Design review of the part built by this model. Coordinates are the model's own, in mm. A direction names the side the tool comes from. Round coordinates to 2 decimals unless told otherwise and drop trailing zeros. Loops run counter-clockwise (first coordinate to the right, second up) from the corner with the lowest first, then second, coordinate; pieces in that order, holes last. Notation, with made-up numbers: M -36.75,81.5 L -3.75,81.5 A31 cw -3.75,107.5 Z; hole C 86,42 d10. An arc over 180 degrees is marked long. One line per item, written item: value. Start each with the question number.
Item 1: For line 1 along X through (y, z) = (1.4, 9); line 2 along Z through (x, y) = (12, 1.55); line 3 along Y through (x, z) = (0, 0.5), list the stretches that pass through material, from the lowest coordinate up.
Item 2: Mouldability with a two-part tool opening along Z and no side actions: class faces 6 (the flat face through (2, 24, -7.75)), 7 (the cylindrical face through (0.35, 8.94, -2.7)), 8 (the cylindrical face through (-13.08, 0.99, -10.18)), 9 (the flat face through (0, 1, 15)) as released by +Z, released by -Z, zero draft, split by the parting line, or undercut.
Item 3: We need section D-D (z = 9). Write out the cut boundary in (x, y), then the cut area to 3 significant figures.
Item 4: We need section A-A (x = 0). State how many separate pieces and enclosed holes the cut face has, then the cut area to 3 significant figures.
Item 5: Clearance check with flat-ended pins moving along their axes: pin 1 (4 mm diameter, centred on x = 6.5, z = -0.5, fed in from -Y); pin 2 (14.5 mm diameter, centred on x = 2.5, y = 22.5, fed in from +Z); pin 3 (11 mm diameter, centred on y = 42, z = 0, fed in from -X); pin 4 (5 mm diameter, centred on x = -12, z = -9, fed in from +Y). State where each tip first meets the part, or that it passes through.
Item 6: We need section B-B (y = 18.5). Write out the cut boundary in (x, z).
Item 7: For faces 1 (the flat face through (0, 58, -10)), 2 (the flat face through (-9, 29, -6)), 3 (the flat face through (0, 2, 10)), 4 (the cylindrical face through (0.1, 6.5, -11.4)), 5 (the flat face through (9, 29, -6)), list the 3-axis set-ups (+Z, -Z, +X, -X, +Y, -Y) from which the entire face can be reached by the end or side of a thin tool; tool diameter is ignored.
Item 8: We need section C-C (x = 12). Write out the cut boundary in (y, z).
Autodesk Inventor part; units mm, degrees
ref_plane "YZ Plane" through (0, 0, 0) normal (1, 0, 0) x (0, 1, 0)
ref_plane "XZ Plane" through (0, 0, 0) normal (0, 1, 0) x (-1, 0, 0)
ref_plane "XY Plane" through (0, 0, 0) normal (0, 0, 1) x (1, 0, 0)
sketch "Sketch1" plane through (0, 0, 0) normal (0, 1, 0) x (-1, 0, 0)
  line L0 (-17, -15) -> (17, -15)
  line L1 (17, -15) -> (17, 15)
  line L2 (17, 15) -> (-17, 15)
  line L3 (-17, 15) -> (-17, -15)
  line L4 (-17, -15) -> (17, 15) construction
  line L5 (17, -15) -> (-17, 15) construction
  point P0 (0, 0)
  dimension "d0" = 34
  dimension "d1" = 30
extrude "Extrusion1" add sketch "Sketch1" along normal blind 2
sketch "Sketch2" plane through (0, 2, 0) normal (0, 1, 0) x (1, 0, 0)
  line L0 (-17, 15) -> (-17, -15)
  line L1 (-17, -15) -> (17, -15)
  line L2 (17, -15) -> (17, 15)
  line L3 (17, 15) -> (-17, 15)
  line L4 (-12, 9) -> (-12, -9) construction
  line L5 (-12, -9) -> (12, -9) construction
  line L6 (12, -9) -> (12, 9) construction
  line L7 (-12, 0) -> (0, 0) construction
  line L8 (0, 0) -> (0, -9) construction
  dimension "d5" = 24
  dimension "d6" = 18
hole "Hole1" at (-12, 2, -9) at (-12, 2, 9) at (12, 2, 9) at (12, 2, -9) direction (0, -1, 0) diameter 3.2 end through all
sketch "Sketch3" plane through (0, 2, 0) normal (0, 1, 0) x (1, 0, 0)
  circle A0 centre (12, 9) radius 1.6
  circle A1 centre (12, -9) radius 1.6
  circle A2 centre (-12, -9) radius 1.6
  circle A3 centre (-12, 9) radius 1.6
  line L0 (-17, 15) -> (-17, -15)
  line L1 (-17, -15) -> (17, -15)
  line L2 (17, -15) -> (17, 15)
  line L3 (17, 15) -> (-17, 15)
  line L4 (-17, -2.5) -> (17, -2.5)
  circle A4 centre (-12, 9) radius 3
  circle A5 centre (12, 9) radius 3
  line L5 (-9, 15) -> (-9, -15)
  line L6 (9, 15) -> (9, -15)
  point P0 (0, 0)
  point P1 (9, -2.5)
  point P2 (-9, -2.5)
  dimension "d14" = 17.5
  dimension "d15" = 6
  dimension "d16" = 8
  dimension "d17" = 8
extrude "Extrusion2" add sketch "Sketch3" along normal blind 30 contours L3 L6 L4 L5
sketch "Sketch4" plane through (17, 0, -15) normal (0, 0, -1) x (-1, 0, 0)
  line L0 (0, 0) -> (34, 0)
  line L1 (34, 0) -> (34, 2)
  line L2 (26, 2) -> (34, 2)
  line L3 (26, 2) -> (26, 32)
  line L4 (8, 32) -> (26, 32)
  line L5 (8, 2) -> (8, 32)
  line L6 (0, 2) -> (8, 2)
  line L7 (0, 0) -> (0, 2)
  circle A0 centre (17, 18.5) radius 5.5
  line L8 (17, 18.5) -> (17, 0) construction
  circle A1 centre (17, 18.5) radius 12
  line L9 (17, 18.5) -> (17, 26.5) construction
  circle A2 centre (17, 10.5) radius 1.6
  circle A3 centre (17, 26.5) radius 1.6
  point P0 (26, 26.4373)
  point P1 (8, 26.4373)
  point P2 (8, 10.5627)
  point P3 (26, 10.5627)
  dimension "d20" = 18.5
  dimension "d21" = 24
  dimension "d22" = 11
  dimension "d24" = 8
  dimension "d29" = 3.2
  dimension "d30" = 8
extrude "Extrusion3" cut sketch "Sketch4" against normal blind 7.25 contours L5 A1 L3 | A0 | A2 | A3
extrude "Extrusion4" cut sketch "Sketch4" against normal through all contours A0 | A2 | A3
sketch "Sketch6" plane through (0, 32, 0) normal (0, 1, 0) x (1, 0, 0)
  line L0 (9, 15) -> (-9, 15)
  line L1 (-9, 15) -> (-9, -2.5)
  line L2 (-9, -2.5) -> (9, -2.5)
  line L3 (9, -2.5) -> (9, 15)
  line L4 (-9, 10) -> (9, 10)
  point P0 (0, 0)
  dimension "d33" = 5
extrude "Extrusion6" add sketch "Sketch6" along normal blind 40 contours L3 L4 L1 L0
chamfer "Chamfer1" distance 12.5 angle 45 1 edges at (0, 32, -10)
chamfer "Chamfer2" distance 5 angle 45 1 edges at (0, 2, 2.5)
equation "\"d17\" = d16"
equation "\"d24\" = d30"
A:
1. line 1: -17 to -13.6, -10.4 to 10.4, 13.6 to 17
1. line 2: -15 to -10.6, -7.4 to 7.4, 10.6 to 15
1. line 3: 0 to 8.9, 12.1 to 13, 24 to 24.9, 28.1 to 34
2. face 6: released by -Z
2. face 7: zero draft
2. face 8: undercut
2. face 9: released by +Z
3. outline: M -17,0 L -13.6,0 L -13.6,2 L -17,2 Z; M -10.4,0 L 10.4,0 L 10.4,2 L -10.4,2 Z; M 13.6,0 L 17,0 L 17,2 L 13.6,2 Z
3. area: 55.2 mm2
4. separate pieces: 4
4. enclosed holes: 0
4. area: 523 mm2
5. pin 1: y = 0
5. pin 2: z = 2.5
5. pin 3: x = -9
5. pin 4: y = 2
6. outline: M -9,-7.75 L -5.5,-7.75 L -5.5,2.5 L -9,2.5 Z; M 5.5,-7.75 L 9,-7.75 L 9,2.5 L 5.5,2.5 Z
7. face 1: +Z, +X, -X, +Y
7. face 2: +Z, -Z, -X, +Y
7. face 3: +Z, +Y
7. face 4: -Z
7. face 5: +Z, -Z, +X, +Y
8. outline: M 0,-15 L 2,-15 L 2,-10.6 L 0,-10.6 Z; M 0,-7.4 L 2,-7.4 L 2,7.4 L 0,7.4 Z; M 0,10.6 L 2,10.6 L 2,15 L 0,15 Z
